```python
from build123d import *

# Parameters (mm, degrees)
SKETCH1_W           = 42
SKETCH1_H           = 42
BOSS_EXTRUDE1_DEPTH = 40
CHAMFER1_SIZE       = 3.5
SKETCH2_R           = 11
BOSS_EXTRUDE2_DEPTH = 2
SKETCH3_R           = 1.5
CUT_EXTRUDE1_DEPTH  = 50.819674828
SKETCH4_R           = 2.5
BOSS_EXTRUDE3_DEPTH = 13
BOSS_EXTRUDE4_START = 15
SKETCH5_R           = 2.5
BOSS_EXTRUDE4_DEPTH = 15
CUT_EXTRUDE2_START  = -3
SKETCH8_R           = 4.5
SKETCH8_R_2         = 2.5
CUT_EXTRUDE2_DEPTH  = 3


with BuildPart() as part:
    # Sketch1 → Boss-Extrude1 (new body)
    with BuildSketch(Plane.XY):
        Rectangle(SKETCH1_W, SKETCH1_H)
    extrude(amount=-BOSS_EXTRUDE1_DEPTH)

    # Chamfer1
    chamfer1_edges = [part.edges().sort_by_distance(p)[0] for p in [
        (21, -21, -20),
        (-21, -21, -20),
        (-21, 21, -20),
        (21, 21, -20),
    ]]
    chamfer(chamfer1_edges, length=CHAMFER1_SIZE)

    # Sketch2 → Boss-Extrude2 (add)
    with BuildSketch(Plane.XY):
        with Locations(Location((0, 0, 0), (0, 0, 180))):
            Circle(SKETCH2_R)
    extrude(amount=BOSS_EXTRUDE2_DEPTH)

    # Sketch3 → Cut-Extrude1 (cut, through all)
    with BuildSketch(Plane.XY):
        with Locations((15.5, 15.5)):
            Circle(SKETCH3_R)
        with Locations((-15.5, 15.5)):
            Circle(SKETCH3_R)
        with Locations((-15.5, -15.5)):
            Circle(SKETCH3_R)
        with Locations((15.5, -15.5)):
            Circle(SKETCH3_R)
    extrude(amount=-CUT_EXTRUDE1_DEPTH, mode=Mode.SUBTRACT)

    # Sketch4 → Boss-Extrude3 (add)
    with BuildSketch(Plane.XY.offset(2)):
        with Locations(Location((0, 0, 0), (0, 0, 180))):
            Circle(SKETCH4_R)
    extrude(amount=BOSS_EXTRUDE3_DEPTH)

    # Sketch5 → Boss-Extrude4 (add)
    with BuildSketch(Plane(origin=(0, 0, -40), x_dir=(-1, 0, 0), z_dir=(0, 0, -1)).offset(BOSS_EXTRUDE4_START)):
        Circle(SKETCH5_R)
    extrude(amount=-BOSS_EXTRUDE4_DEPTH)

    # Sketch8 → Cut-Extrude2 (cut)
    with BuildSketch(Plane.XY.offset(2).offset(CUT_EXTRUDE2_START)):
        Circle(SKETCH8_R)
        with Locations(Location((0, 0, 0), (0, 0, 180))):
            Circle(SKETCH8_R_2, mode=Mode.SUBTRACT)
    extrude(amount=CUT_EXTRUDE2_DEPTH, mode=Mode.SUBTRACT)


solid = part.part
```
Input: part model. Units: mm. Frame: model coordinates. A direction names the side the tool comes from. Give positions to 0.01 mm unless a question says otherwise; leave off trailing zeros. Order: outer loops, then holes, each group sorted by start corner. A loop starts at its lowest first (then second) coordinate and runs counter-clockwise, first axis right, second up. Notation, with made-up numbers: (45, -16) -> (102, -16) arc R29 cw to (102, 23) -> close; hole circle Ø4 at (11, 22). An arc over 180 degrees is marked (long way). Write each question's results on one line, items separated by ' | '. Start each with the question number.
Item 1: Line query: line 1 (Y direction, x = 15.5, z = -17.5); line 2 (Y direction, x = 0, z = 0.5); line 3 (X direction, y = 15, z = -19). Output: solid intervals per line, ascending.
Item 2: Set-up query: faces 4 (the cylindrical face through (-0.59, 4.46, 0.48)), 5 (the flat face through (19.3, -19.2, -19.7)), 6 (the cylindrical face through (0.54, -2.44, -47.6)). Return all of +Z, -Z, +X, -X, +Y, -Y with unobstructed straight access to the full face (end or side cutting, diameter ignored); none if empty.
Item 3: Mould query, pull axis X, two halves, no side actions, for faces 1 (the flat face through (-19.2, 19.3, -19.7)), 2 (the cylindrical face through (-17, 15.57, -19.72)), 3 (the cylindrical face through (2.38, 10.74, 0.99)). Classes: pulls with the +X half, pulls with the -X half, needs draft (parallel to the pull), parting line crosses it, or undercut.
Item 4: Contact query for flat-ended pins moving along their axis: P1, Ø1.5, axis at x = -12, y = -12.5, coming from the -Z side; P2, Ø2.5, axis at x = 15.5, y = 15.5, coming from the +Z side; P3, Ø12, axis at x = -13, y = -16, coming from the +Z side. Output: stop coordinate, or through.
Item 5: Cut plane A-A on y = -15.5. Return the cut outline in (x, z), then the cut area to 3 significant figures.
Item 6: Cut plane C-C on z = -29. Return the cut outline in (x, y), then the cut area to 3 significant figures.
Item 7: Cut plane D-D on x = 0. Return the cut outline in (y, z).
Established:
1) line 1: -21 to -17, -14 to 14, 17 to 21 | line 2: -11 to -4.5, -2.5 to 2.5, 4.5 to 11 | line 3: -21 to -16.91, -14.09 to 14.09, 16.91 to 21
2) face 4: +Z | face 5: +Z, -Z, +X, -Y | face 6: -Z
3) face 1: pulls with the -X half | face 2: undercut | face 3: parting line crosses it
4) P1: z = -40 | P2: through | P3: z = 0
5) outline: (-21, -40) -> (-17, -40) -> (-17, 0) -> (-21, 0) -> close; (-14, -40) -> (14, -40) -> (14, 0) -> (-14, 0) -> close; (17, -40) -> (21, -40) -> (21, 0) -> (17, 0) -> close | area: 1,440 mm^2
6) outline: (-21, -17.5) -> (-17.5, -21) -> (17.5, -21) -> (21, -17.5) -> (21, 17.5) -> (17.5, 21) -> (-17.5, 21) -> (-21, 17.5) -> close; hole circle Ø3 at (-15.5, -15.5); hole circle Ø3 at (-15.5, 15.5); hole circle Ø3 at (15.5, -15.5); hole circle Ø3 at (15.5, 15.5) | area: 1,710 mm^2
7) outline: (-21, -40) -> (-2.5, -40) -> (-2.5, -55) -> (2.5, -55) -> (2.5, -40) -> (21, -40) -> (21, 0) -> (11, 0) -> (11, 2) -> (4.5, 2) -> (4.5, -1) -> (2.5, -1) -> (2.5, 15) -> (-2.5, 15) -> (-2.5, -1) -> (-4.5, -1) -> (-4.5, 2) -> (-11, 2) -> (-11, 0) -> (-21, 0) -> close
